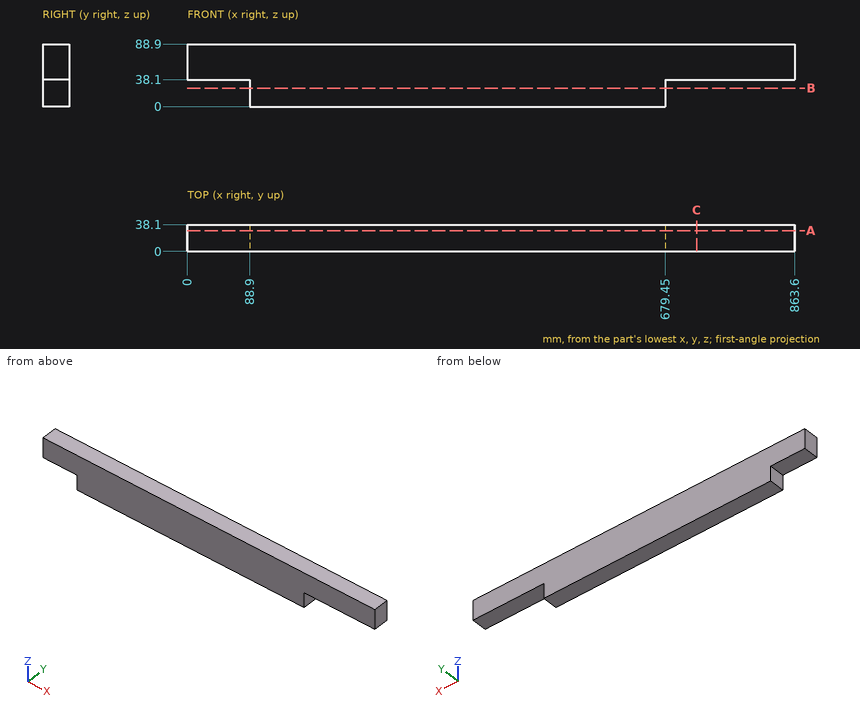
Job drawing, mm, ordinate dimensions from the low corner. One solid piece. Coordinates: 2 decimals unless noted, no trailing zeros. Order: outer loops, then holes, each group sorted by start corner. A loop starts at its lowest first (then second) coordinate and runs counter-clockwise, first axis right, second up. Notation, with made-up numbers: (81.5, 21.25) - (106.5, 21.25) arc R14 ccw to (106.5, 48.25) - close; hole circle Ø8 at (-6.75, -2.5). An arc over 180 degrees is marked (long way). Return JSON: item names as keys, results as strings. Group by question number.
1) Saw through at A-A, the plane y = 29.5. Write the cut outline in (x, z).
2) Probe line 1 (Z direction, x = 741.5, y = 31); line 2 (X direction, y = 14.5, z = 30.5). List the from-to ranges inside material, lowest first. Write a range as from..to.
3) Flat gauge pins, fed straight in: P1, Ø11.5, axis at y = 22, z = 21, coming from the -X side; P2, Ø3, axis at x = 695, y = 24.5, coming from the -Z side. Where does each tip first touch, or does it go through?
4) Saw through at B-B, the plane z = 26. Write the cut outline in (x, y), plus the area to 3 significant figures.
5) Saw through at C-C, the plane x = 724.5. Write the cut outline in (y, z), plus the area to 3 significant figures.
Values found:
{
 "1": {"outline": "(0, 38.1) - (88.9, 38.1) - (88.9, 0) - (679.45, 0) - (679.45, 38.1) - (863.6, 38.1) - (863.6, 88.9) - (0, 88.9) - close"},
 "2": {"line 1": "z = 38.1..88.9", "line 2": "x = 88.9..679.45"},
 "3": {"P1": "stops at x = 88.9", "P2": "stops at z = 38.1"},
 "4": {"outline": "(88.9, 0) - (679.45, 0) - (679.45, 38.1) - (88.9, 38.1) - close", "area": "22,500 mm²"},
 "5": {"outline": "(0, 38.1) - (38.1, 38.1) - (38.1, 88.9) - (0, 88.9) - close", "area": "1,940 mm²"}
}
